Read the model definition and answer for the solid it produces. Units are mm, in the model's axes. Face numbers are marked on the shaded views. A direction names the side the tool comes from. Round coordinates to 2 decimals unless told otherwise and drop trailing zeros. Order: outer loops, then holes, each group sorted by start corner. A loop starts at its lowest first (then second) coordinate and runs counter-clockwise, first axis right, second up. Notation, with made-up numbers: (53, 6.5) - (81, 6.5) arc R30 cw to (81, 39.5) - close; hole circle Ø3 at (35, 10). An arc over 180 degrees is marked (long way). One line per question, with ' | ' between items. Start each with the question number.
1) The part is cut by section B-B, the plane z = 0. Give the vertices of the cut face in (x, y).
2) Straight lines are drawn through the part: line 1 (X direction, y = 0, z = -0.1); line 2 (Y direction, x = 0.9, z = 2); line 3 (Z direction, x = 0.1, y = 2.25). For each, find the intervals that lie inside material, in ascending order. Write a range as from..to.
3) The part is cut by section D-D, the plane y = 3.25. Give the vertices of the cut face in (x, z).
4) The part is cut by section C-C, the plane y = 1. Give the vertices of the cut face in (x, z).
5) For the marked faces 1, 2 and 3, determine the directions among +Z, -Z, +X, -X, +Y, -Y from which every point of the face is accessible in a straight line to the end or side of a thin tool.
6) The part is cut by section A-A, the plane x = 0. Give the vertices of the cut face in (y, z).
from build123d import *

# Parameters (mm, degrees)
SKETCH1_R           = 2.286
BOSS_EXTRUDE1_DEPTH = 1.5875
SKETCH2_R           = 1.524
BOSS_EXTRUDE2_DEPTH = 3.556


with BuildPart() as part:
    # Sketch1 → Boss-Extrude1 (new body, symmetric)
    with BuildSketch(Plane(origin=(0, 0, 0), x_dir=(1, 0, 0), z_dir=(0, 1, 0))):
        Circle(SKETCH1_R)
    extrude(amount=BOSS_EXTRUDE1_DEPTH, both=True)

    # Sketch2 → Boss-Extrude2 (add)
    with BuildSketch(Plane(origin=(0, -1.5875, 0), x_dir=(-1, 0, 0), z_dir=(0, -1, 0))):
        Circle(SKETCH2_R)
    boss_extrude2 = extrude(amount=BOSS_EXTRUDE2_DEPTH)

    # Mirror1: Boss-Extrude2 across plane
    add(boss_extrude2.mirror(Plane.ZX))


solid = part.part
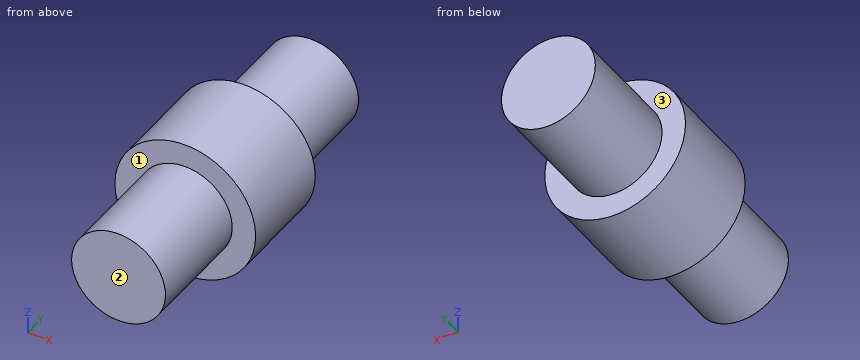
Values:
1) outline: (-2.29, -1.59) - (-1.52, -1.59) - (-1.52, -5.14) - (1.52, -5.14) - (1.52, -1.59) - (2.29, -1.59) - (2.29, 1.59) - (1.52, 1.59) - (1.52, 5.14) - (-1.52, 5.14) - (-1.52, 1.59) - (-2.29, 1.59) - close
2) line 1: x = -2.28..2.28 | line 2: y = -1.59..1.59 | line 3: z = -1.52..1.52
3) outline: circle Ø3.05 at (0, 0)
4) outline: circle Ø4.57 at (0, 0)
5) face 1: -Y | face 2: +Z, -Z, +X, -X, -Y | face 3: +Y
6) outline: (-5.14, -1.52) - (-1.59, -1.52) - (-1.59, -2.29) - (1.59, -2.29) - (1.59, -1.52) - (5.14, -1.52) - (5.14, 1.52) - (1.59, 1.52) - (1.59, 2.29) - (-1.59, 2.29) - (-1.59, 1.52) - (-5.14, 1.52) - close
